Part print with two shaded views. Sizes in mm from the minimum x, y, z corner. A direction names the side the tool comes from. Round coordinates to 2 decimals unless told otherwise and drop trailing zeros. Write each loop counter-clockwise with the first axis right and the second up, starting at its lowest first coordinate (ties: lowest second). Pieces come first, ordered by that corner, then holes. Notation, with made-up numbers: (2, 66) -> (47, 66) arc R32 ccw to (47, 94) -> close; hole circle Ø3 at (86.5, 83.5). An arc over 180 degrees is marked (long way). Answer as CSV lines item,"result".
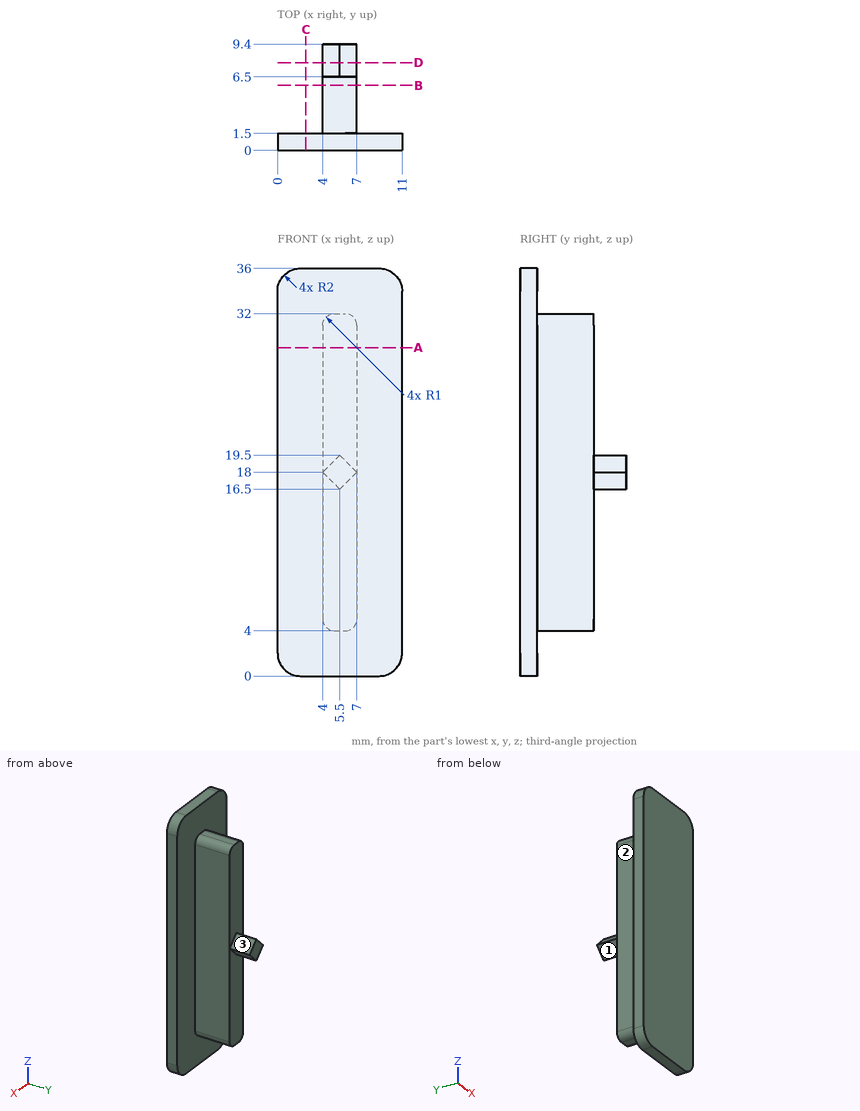
1. Cut at B-B, the plane y = 5.75. Write the cut outline in (x, z), then the cut area to 3 significant figures.
Results found:
outline,"(4, 5) arc R1 ccw to (5, 4) -> (6, 4) arc R1 ccw to (7, 5) -> (7, 31) arc R1 ccw to (6, 32) -> (5, 32) arc R1 ccw to (4, 31) -> close"
area,"83.1 mm2"
2. Probe line 1 along Y through (x, z) = (6, 14); line 2 along Z through (x, y) = (5.25, 5); line 3 along X through (y, z) = (2.5, 9). List the from-to ranges inside material, lowest first.
Results found:
line 1,"y = 0 to 6.5"
line 2,"z = 4 to 32"
line 3,"x = 4 to 7"
3. Cut at C-C, the plane x = 2.5. Write the cut outline in (y, z).
Results found:
outline,"(0, 0) -> (1.5, 0) -> (1.5, 36) -> (0, 36) -> close"
4. Drop flat-ended pins along their axis: pin 1 Ø0.5 at (x, y) = (5.5, 4) entering from -Z; pin 2 Ø2 at (x, y) = (7.5, 3) entering from +Z; pin 3 Ø1.5 at (x, z) = (3.5, 8.5) entering from +Y; pin 4 Ø6 at (x, z) = (2.5, 10.5) entering from -Y. Give the stop position or say it passes through.
Results found:
pin 1,"stops at z = 4"
pin 2,"stops at z = 31.87"
pin 3,"stops at y = 6.5"
pin 4,"stops at y = 0"
5. Cut at D-D, the plane y = 7.75. Write the cut outline in (x, z), then the cut area to 3 significant figures.
Results found:
outline,"(4, 18) -> (5.5, 16.5) -> (7, 18) -> (5.5, 19.5) -> close"
area,"4.50 mm2"
6. Cut at A-A, the plane z = 29. Write the cut outline in (x, y).
Results found:
outline,"(0, 0) -> (11, 0) -> (11, 1.5) -> (7, 1.5) -> (7, 6.5) -> (4, 6.5) -> (4, 1.5) -> (0, 1.5) -> close"
7. Which spindle directions (+Z, -Z, +X, -X, +Y, -Y) get a long thin tool onto all of the face, cutting with end or side? Do the marked faces 1, 2 and 3. Say none if no direction does.
Results found:
face 1,"-Z, -X, +Y"
face 2,"+Z, -Z, -X, +Y"
face 3,"+Z, +X, +Y"
